Design review of the part built by this model. Coordinates are the model's own, in mm. Face numbers are marked on the shaded views. Coordinates: 2 decimals unless noted, no trailing zeros. Order: outer loops, then holes, each group sorted by start corner. A loop starts at its lowest first (then second) coordinate and runs counter-clockwise, first axis right, second up.
from build123d import *

# Parameters (mm, degrees)
CROQUIS1_W              = 250
CROQUIS1_H              = 221
SALIENTE_EXTRUIR1_DEPTH = 5.5
SALIENTE_EXTRUIR2_DEPTH = 15
CROQUIS3_W              = 150
CROQUIS3_H              = 100
SALIENTE_EXTRUIR3_DEPTH = 15
FILLET1_R               = 5


with BuildPart() as part:
    # Croquis1 → Saliente-Extruir1 (new body)
    with BuildSketch(Plane(origin=(0, 0, 0), x_dir=(1, 0, 0), z_dir=(0, 1, 0))):
        Rectangle(CROQUIS1_W, CROQUIS1_H)
    extrude(amount=SALIENTE_EXTRUIR1_DEPTH)

    # Croquis2 → Saliente-Extruir2 (add)
    with BuildSketch(Plane.XZ):
        Polygon((-125, 110.5), (-100, 110.5), (-100, 90.5), (-105, 90.5), (-105, 85.5), (-125, 85.5), align=None)
        Polygon((125, -110.5), (125, -85.5), (105, -85.5), (105, -90.5), (100, -90.5), (100, -110.5), align=None)
    saliente_extruir2 = extrude(amount=SALIENTE_EXTRUIR2_DEPTH)

    # Simetría1: Saliente-Extruir2 across plane
    add(saliente_extruir2.mirror(Plane.XY))

    # Croquis3 → Saliente-Extruir3 (add)
    with BuildSketch(Plane.XZ):
        Rectangle(CROQUIS3_W, CROQUIS3_H)
    extrude(amount=SALIENTE_EXTRUIR3_DEPTH)

    # Fillet1
    fillet1_edges = [part.edges().sort_by_distance(p)[0] for p in [
        (125, -4.75, 110.5),
        (-125, -4.75, 110.5),
        (-125, -4.75, -110.5),
        (125, -4.75, -110.5),
    ]]
    fillet(fillet1_edges, radius=FILLET1_R)


solid = part.part
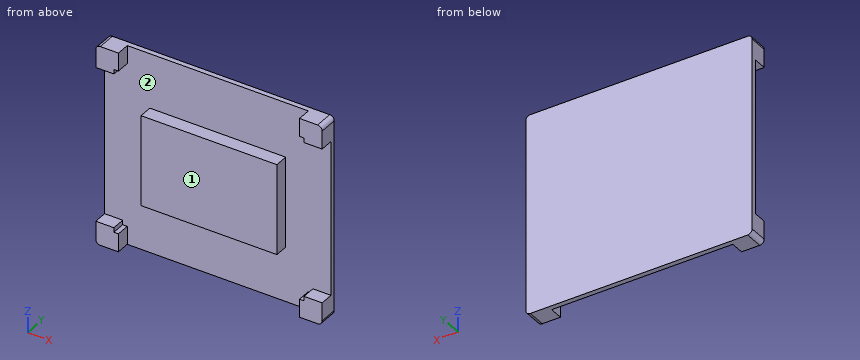
1. Add section A-A (y = -3.25). State how many separate pieces and enclosed holes the cut face has, and give its area (3 significant figures).
2. Add section B-B (z = -10). Give the boundary of the cut face in (x, y).
3. Insertion check: pin 1 (7.5 mm diameter, centred on y = -6, z = 5.5, fed in from +X); pin 2 (4 mm diameter, centred on x = 62, y = -4.5, fed in from -Z); pin 3 (1 mm diameter, centred on x = -34.5, y = -1.5, fed in from +Z). Each pin has a flat end and moves straight along its axis. Give the tip position at first contact, or say it passes through.
4. To check wall thickness, follow line 1 (X direction, y = -5.75, z = -95); line 2 (Z direction, x = -110, y = -8.75); line 3 (Y direction, x = -83, z = 25). State the ranges of each line that lie inside material, in increasing order.
5. Add section C-C (x = -0.5). Give the boundary of the cut face in (y, z), and give its area (3 significant figures).
6. Mouldability with a two-part tool opening along X and no side actions: class the marked faces 1 and 2 as pulls with the +X half, pulls with the -X half, needs draft (parallel to the pull), parting line crosses it, or undercut.
7. Add section D-D (z = 69.5). Give the boundary of the cut face in (x, y).
Solution:
1. separate pieces: 5
1. enclosed holes: 0
1. area: 17,400 mm2
2. outline: (-125, 0) - (-75, 0) - (-75, -15) - (75, -15) - (75, 0) - (125, 0) - (125, 5.5) - (-125, 5.5) - close
3. pin 1: stops at x = 75
3. pin 2: stops at z = -50
3. pin 3: stops at z = 50
4. line 1: x = -125 to -100, 100 to 125
4. line 2: z = -110.5 to -85.5, 85.5 to 110.5
4. line 3: y = 0 to 5.5
5. outline: (-15, -50) - (0, -50) - (0, -110.5) - (5.5, -110.5) - (5.5, 110.5) - (0, 110.5) - (0, 50) - (-15, 50) - close
5. area: 2,720 mm2
6. face 1: needs draft
6. face 2: undercut
7. outline: (-125, 0) - (125, 0) - (125, 5.5) - (-125, 5.5) - close
